```python
from build123d import *

# Parameters (mm, degrees)
SKETCH_1_R          = 1.5
SKETCH_1_R_2        = 1.75
EXTRUDE_1_DEPTH     = 3
FILLET_1_R          = 5
SKETCH_2_R          = 0.5
CUT_EXTRUDE_1_DEPTH = 10
FILLET_2_R          = 2
SKETCH_3_R          = 4.05
CUT_EXTRUDE_2_DEPTH = 10
FILLET_3_R          = 1


with BuildPart() as part:
    # 草图1 → 凸台-拉伸1 (new body)
    with BuildSketch(Plane(origin=(0, 0, 0), x_dir=(0, 0, -1), z_dir=(1, 0, 0))):
        with BuildLine():
            Line((-48, -20.45), (-48, -28.65))
            Line((-48, -28.65), (-52, -28.65))
            Line((-52, -28.65), (-52, -56.25))
            Line((-52, -56.25), (15.786547457, -56.25))
            Line((15.786547457, -56.25), (48.25, -17.561563803))
            Line((48.25, -17.561563803), (48.25, -10))
            Line((48.25, -10), (33.25, -10))
            Line((33.25, -10), (28.415845032, -17.74231527))
            ThreePointArc((28.415845032, -17.74231527), (-8.807963632, -32.321351714), (-33.488633754, -0.872587709))
            Line((-33.488633754, -0.872587709), (-43.660254038, 5))
            Line((-43.660254038, 5), (-60, 5))
            Line((-60, 5), (-60, -20.45))
            Line((-60, -20.45), (-48, -20.45))
        make_face()
        with Locations((-45, -51.25)):
            Circle(SKETCH_1_R, mode=Mode.SUBTRACT)
        with Locations((-10, -51.25)):
            Circle(SKETCH_1_R, mode=Mode.SUBTRACT)
        with Locations((-30.0520382, -30.0520382)):
            Circle(SKETCH_1_R_2, mode=Mode.SUBTRACT)
        with Locations((10, -51.25)):
            Circle(SKETCH_1_R, mode=Mode.SUBTRACT)
        with Locations((0, -42.5)):
            Circle(SKETCH_1_R_2, mode=Mode.SUBTRACT)
        with Locations((30.0520382, -30.0520382)):
            Circle(SKETCH_1_R_2, mode=Mode.SUBTRACT)
        with Locations((-55, -15.45)):
            Circle(SKETCH_1_R, mode=Mode.SUBTRACT)
        with Locations((-55, -0.45)):
            Circle(SKETCH_1_R, mode=Mode.SUBTRACT)
        with Locations((-42.5, 0)):
            Circle(SKETCH_1_R_2, mode=Mode.SUBTRACT)
    extrude(amount=EXTRUDE_1_DEPTH)

    # 圆角1
    fillet_1_edges = [part.edges().sort_by_distance(p)[0] for p in [
        (1.5, -10, -33.25),
        (1.5, -17.561563803, -48.25),
        (1.5, 5, 43.660254038),
        (1.5, -0.872587709, 33.488633754),
    ]]
    fillet(fillet_1_edges, radius=FILLET_1_R)

    # 草图2 → 切除-拉伸1 (cut)
    with BuildSketch(Plane.ZY):
        with Locations((48, -20.45)):
            Circle(SKETCH_2_R)
        with Locations((48, -28.65)):
            Circle(SKETCH_2_R)
    extrude(amount=-CUT_EXTRUDE_1_DEPTH, mode=Mode.SUBTRACT)

    # 圆角2
    fillet_2_edges = [part.edges().sort_by_distance(p)[0] for p in [
        (1.5, -10, -48.25),
    ]]
    fillet(fillet_2_edges, radius=FILLET_2_R)

    # 草图3 → 切除-拉伸2 (cut)
    with BuildSketch(Plane.ZY):
        with Locations((19, -48.75)):
            Circle(SKETCH_3_R)
    extrude(amount=-CUT_EXTRUDE_2_DEPTH, mode=Mode.SUBTRACT)

    # 圆角3
    fillet_3_edges = [part.edges().sort_by_distance(p)[0] for p in [
        (1.5, -56.25, -15.786547457),
        (1.5, -56.25, 52),
        (1.5, -28.65, 52),
        (1.5, -20.45, 60),
        (1.5, 5, 60),
    ]]
    fillet(fillet_3_edges, radius=FILLET_3_R)


solid = part.part
```
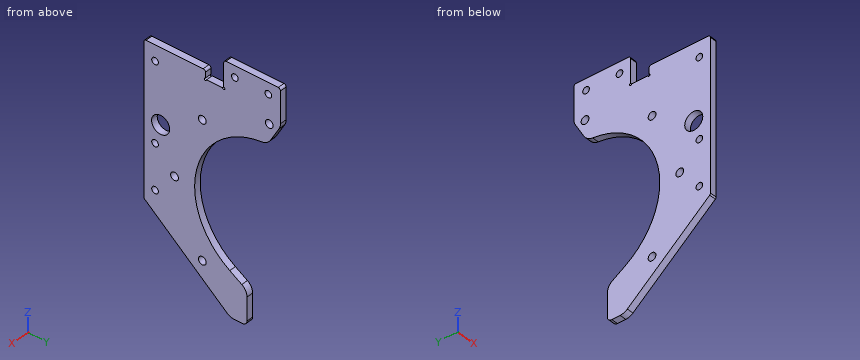
Here's how the part is built. I have some questions about the finished solid (model axes, mm). Round coordinates to 2 decimals unless told otherwise and drop trailing zeros. Order: outer loops, then holes, each group sorted by start corner. A loop starts at its lowest first (then second) coordinate and runs counter-clockwise, first axis right, second up. Notation, with made-up numbers: M 71,-13 L 119,-13 A20 ccw 119,17 Z; hole C -31.75,-35 d7. An arc over 180 degrees is marked long. One line per question, with ' | ' between items.
1) For pin 1 Ø5 at (y, z) = (-51.25, 45) entering from -X; pin 2 Ø1 at (x, y) = (0.5, -43) entering from -Z; pin 3 Ø1 at (x, z) = (0.5, -23.5) entering from +Y; pin 4 Ø0.9 at (x, y) = (1.5, -23.5) entering from +Z, each with a flat end and sliding along its axis, tell me the tip position at first contact or that it passes through.
Working result:
pin 1: x = 0 | pin 2: z = -27.32 | pin 3: y = -23.37 | pin 4: z = 48
2) I want a section at A-A, the plane z = 55. Write out the boundary of the cut face in (x, y).
Working result:
outline: M 0,-20.45 L 3,-20.45 L 3,-16.95 L 0,-16.95 Z; M 0,-13.95 L 3,-13.95 L 3,-1.95 L 0,-1.95 Z; M 0,1.05 L 3,1.05 L 3,5 L 0,5 Z
3) I want a section at C-C, the plane z = 10. Write out the boundary of the cut face in (x, y).
Working result:
outline: M 0,-56.25 L 3,-56.25 L 3,-52.75 L 0,-52.75 Z; M 0,-49.75 L 3,-49.75 L 3,-31.97 L 0,-31.97 Z
4) I need wall thicknesses on line 1 along Z through (x, y) = (1.95, -14.5); line 2 along Y through (x, z) = (1.75, 55); line 3 along Z through (x, y) = (1.35, -29.5). Which ranges of each line are inside material? Lowest first, please.
Working result:
line 1: -48.25 to -30.44, 30.2 to 53.84, 56.16 to 60 | line 2: -20.45 to -16.95, -13.95 to -1.95, 1.05 to 5 | line 3: -38.23 to -31.71, -28.39 to -15.87, 15.87 to 28.39, 31.71 to 51.99
5) I want a section at D-D, the plane x = 2.15. State how many separate pieces and enclosed holes the cut face has, then the cut area to 3 significant figures.
Working result:
separate pieces: 1 | enclosed holes: 10 | area: 3,190 mm²
6) I want a section at B-B, the plane y = -27. Write out the boundary of the cut face in (x, z).
Working result:
outline: M 0,-40.33 L 3,-40.33 L 3,-19.83 L 0,-19.83 Z; M 0,19.83 L 3,19.83 L 3,48 L 0,48 Z
